Geometry check sheet. Reference: the model listing, model coordinates, mm. Round coordinates to 2 decimals unless told otherwise and drop trailing zeros.
```python
from build123d import *

# Parameters (mm, degrees)
F0_W        = 21.5
F0_H        = 21.5
F0_W_2      = 5.5
F0_H_2      = 5.5
F0_W_3      = 3
F0_H_3      = 3
F1_DEPTH    = 3
F2_R        = 2.99999
F3_T1_DEPTH = 51.4949074278
F4_T1_DEPTH = 46.5959279422


# Not quite as in the source:
# - a fillet or chamfer that OpenCascade refuses, or shapes differently, is made with other operations: its cross-section is extruded or revolved along the edge and cut away or added
# - a fillet or chamfer is up to 0.001 mm smaller than in the source, because OpenCascade refuses the exact size


with BuildPart() as f1:
    # F0 (on Front) → F1 (new body)
    with BuildSketch(Plane.XZ):
        with Locations((16.25, 13.75)):
            Rectangle(F0_W, F0_H)
        with BuildLine():
            ThreePointArc((11.4712772337, 8.9712772337), (12.1660339017, 7.9315004007), (12.41, 6.705))
            ThreePointArc((12.41, 6.705), (6.2439660983, 5.4784995993), (11.4712772337, 8.9712772337))
        make_face(mode=Mode.SUBTRACT)
        with BuildLine():
            ThreePointArc((26.5, 6.705), (22.0684995993, 3.7439660983), (21.0287227663, 8.9712772337))
            ThreePointArc((21.0287227663, 8.9712772337), (24.5215004007, 9.6660339017), (26.5, 6.705))
        make_face(mode=Mode.SUBTRACT)
        with BuildLine():
            ThreePointArc((18.5162772337, 11.4837227663), (16.25, 10.545), (13.9837227663, 11.4837227663))
            ThreePointArc((13.9837227663, 11.4837227663), (13.045, 13.75), (13.9837227663, 16.0162772337))
            ThreePointArc((13.9837227663, 16.0162772337), (16.25, 16.955), (18.5162772337, 16.0162772337))
            ThreePointArc((18.5162772337, 16.0162772337), (19.2110339017, 14.9765004007), (19.455, 13.75))
            ThreePointArc((19.455, 13.75), (19.2110339017, 12.5234995993), (18.5162772337, 11.4837227663))
        make_face(mode=Mode.SUBTRACT)
        with BuildLine():
            ThreePointArc((12.41, 20.795), (12.1660339017, 19.5684995993), (11.4712772337, 18.5287227663))
            ThreePointArc((11.4712772337, 18.5287227663), (6.2439660983, 22.0215004007), (12.41, 20.795))
        make_face(mode=Mode.SUBTRACT)
        with BuildLine():
            ThreePointArc((26.5, 20.795), (24.5215004007, 17.8339660983), (21.0287227663, 18.5287227663))
            ThreePointArc((21.0287227663, 18.5287227663), (22.0684995993, 23.7560339017), (26.5, 20.795))
        make_face(mode=Mode.SUBTRACT)
        with Locations((2.75, 13.75)):
            Rectangle(F0_W_2, F0_H)
        with Locations((2.75, 27.25)):
            Rectangle(F0_W_2, F0_H_2)
        with Locations((16.25, 27.25)):
            Rectangle(F0_W, F0_H_2)
        with Locations((28.5, 27.25)):
            Rectangle(F0_W_3, F0_H_2)
        with Locations((28.5, 13.75)):
            Rectangle(F0_W_3, F0_H)
        with BuildLine():
            Line((27, 3), (27, 0))
            ThreePointArc((27, 0), (29.1213203436, 0.8786796564), (30, 3))
            Line((30, 3), (27, 3))
        make_face()
        with Locations((16.25, 1.5)):
            Rectangle(F0_W, F0_H_3)
        with Locations((2.75, 1.5)):
            Rectangle(F0_W_2, F0_H_3)
    extrude(amount=F1_DEPTH)

    # F2 (radius 3 in the source; OpenCascade refuses exactly that, so slightly less here)
    f2_edges = [f1.edges().sort_by_distance(p)[0] for p in [
        (29.12132, -3, 0.87868),
        (13.5, -3, 0),
        (30, -3, 16.5),
    ]]
    fillet(f2_edges, radius=F2_R)

    # F3: fillet of radius 5.5 on 1 edges, made by hand

    # F3_s2 → F3_t1 (cut)
    with BuildSketch(Plane.XY.offset(-9.2474587139)):
        with BuildLine():
            ThreePointArc((4.8989794856, -3), (2.0266981623, -2.1904157598), (0, 0))
            Line((0, 0), (0, -3))
            Line((0, -3), (4.8989794856, -3))
        make_face()
    extrude(amount=F3_T1_DEPTH, mode=Mode.SUBTRACT)

    # F4: fillet of radius 5.5 on 1 edges, made by hand

    # F4_s2 → F4_t1 (cut)
    with BuildSketch(Plane.YZ.offset(-7.3484692283)):
        with BuildLine():
            ThreePointArc((0, 30), (-2.1904157598, 27.9733018377), (-3, 25.1010205144))
            Line((-3, 25.1010205144), (-3, 30))
            Line((-3, 30), (0, 30))
        make_face()
    extrude(amount=F4_T1_DEPTH, mode=Mode.SUBTRACT)


solid = f1.part
```
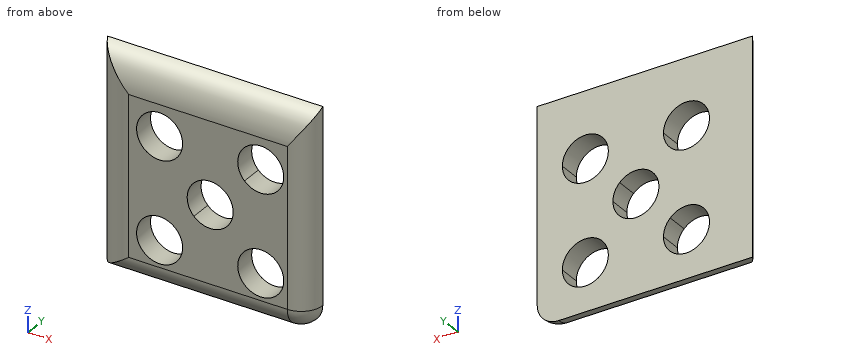
1) Scan lines: line 1 along X through (y, z) = (-2.5, 23); line 2 along X through (y, z) = (-0.4, 23); line 3 along Z through (x, y) = (21, -0.45). Record each from-to range of solid material in increasing order.
Report:
line 1: x = 2.61 to 6.88, 11.53 to 20.97, 25.62 to 28.66
line 2: x = 0.23 to 6.88, 11.53 to 20.97, 25.62 to 29.97
line 3: z = 0.03 to 4.47, 8.94 to 18.56, 23.03 to 29.74
2) Sectioned sample at A-A, the plane x = 20.5. State how many separate pieces and enclosed holes the cut face has, then the cut area to 3 significant figures.
Report:
separate pieces: 3
enclosed holes: 0
area: 65.0 mm2
3) Gauge pin test, flat ends, axial feed: pin 1 (1.5 mm diameter, centred on x = 26, y = -1.5, fed in from -Z); pin 2 (5 mm diameter, centred on x = 23.295, z = 20.795, fed in from +Y). Record the tip position at first contact, or that the pin passes through.
Report:
pin 1: stops at z = 0.1
pin 2: passes through
